from build123d import *

# Parameters (mm, degrees)
F0_W      = 50
F0_H      = 100
F1_DEPTH  = 20
F2_R      = 10
F3_DEPTH  = 10
F4_R      = 5
F5_DEPTH  = 10
F6_R      = 5
F7_DEPTH  = 10
F8_W      = 50
F8_H      = 10
F9_DEPTH  = 110
F10_R     = 10
F12_DEPTH = 10


with BuildPart() as f1:
    # F0 (on Top) → F1 (new body)
    with BuildSketch(Plane.XY):
        with Locations((25, 50)):
            Rectangle(F0_W, F0_H)
    extrude(amount=F1_DEPTH)

    # F2 (on face) → F3 (cut)
    with BuildSketch(Plane.XY.offset(20)):
        with Locations((25, 75)):
            Circle(F2_R)
        with Locations((25, 40)):
            Circle(F2_R)
    extrude(amount=-F3_DEPTH, mode=Mode.SUBTRACT)

    # F4 (on face) → F5 (cut)
    with BuildSketch(Plane.XY.offset(10)):
        with Locations((25, 75)):
            Circle(F4_R)
    extrude(amount=-F5_DEPTH, mode=Mode.SUBTRACT)

    # F6 (on face) → F7 (cut)
    with BuildSketch(Plane.XY.offset(10)):
        with Locations((25, 40)):
            Circle(F6_R)
    extrude(amount=-F7_DEPTH, mode=Mode.SUBTRACT)

    # F8 (on face) → F9 (join)
    with BuildSketch(Plane.XY.offset(20)):
        with Locations((25, 5)):
            Rectangle(F8_W, F8_H)
    extrude(amount=F9_DEPTH)

    # F10
    f10_edges = [f1.edges().sort_by_distance(p)[0] for p in [
        (0, 100, 10),
        (50, 100, 10),
        (0, 5, 130),
        (50, 5, 130),
    ]]
    fillet(f10_edges, radius=F10_R)

    # F11 (on face) → F12 (cut)
    with BuildSketch(Plane(origin=(0, 10, 0), x_dir=(-1, 0, 0), z_dir=(0, 1, 0))):
        with BuildLine():
            Line((-33, 105), (-33, 40))
            ThreePointArc((-33, 40), (-25, 32), (-17, 40))
            Line((-17, 40), (-17, 105))
            ThreePointArc((-17, 105), (-25, 113), (-33, 105))
        make_face()
    extrude(amount=-F12_DEPTH, mode=Mode.SUBTRACT)


solid = f1.part
Input: part model. Units: mm. Frame: model coordinates. A direction names the side the tool comes from. Give positions to 0.01 mm unless a question says otherwise; leave off trailing zeros. Write each loop counter-clockwise with the first axis right and the second up, starting at its lowest first coordinate (ties: lowest second). Pieces come first, ordered by that corner, then holes. Notation, with made-up numbers: (74, 18.25) -> (123, 18.25) arc R15 ccw to (123, 35.25) -> close; hole circle Ø1 at (56.5, -25.75). An arc over 180 degrees is marked (long way). Use one line per item in the form item = value. Start each with the question number.
1) Pin query (flat end, axial travel): pin 1 (1 mm diameter, centred on x = 31, z = 106, fed in from -Y); pin 2 (12 mm diameter, centred on x = 25, y = 40, fed in from +Z); pin 3 (4 mm diameter, centred on x = 35.5, z = 106.5, fed in from +Y); pin 4 (16 mm diameter, centred on x = 23.5, y = 77, fed in from +Z). Return the tip coordinate at first contact, or that it passes through.
2) Section query B-B on y = 40. Return the cut outline in (x, z).
3) Draft query along X for faces 5 (the cylindrical face through (25, 5, 113)), 6 (the cylindrical face through (47.15, 96.99, 10.14)), 7 (the cylindrical face through (2.85, 96.99, 10.14)). Return one class per face: pulls with the +X half, pulls with the -X half, needs draft (parallel to the pull), parting line crosses it, or undercut.
4) Set-up query: faces 1 (the flat face through (25, 56, 20)), 2 (the flat face through (20, 73, 10)), 3 (the flat face through (33, 5, 73)), 4 (the flat face through (25, 5, 130)). Return all of +Z, -Z, +X, -X, +Y, -Y with unobstructed straight access to the full face (end or side cutting, diameter ignored); none if empty.
5) Section query D-D on x = 8.5. Return the cut outline in (y, z), then the cut area to 3 significant figures.
6) Ray query, probe 1 along Y at (x, z) = (25, 14.75); probe 2 along Y at (x, z) = (25, 5); probe 3 along Z at (x, y) = (14, 63). Return the intervals inside material, ascending. Write a range as from..to.
7) Section query C-C on z = 16.5. Return the cut outline in (x, y).
8) Section query A-A on z = 90. Return the cut outline in (x, y).
Outcome:
q1.pin_1 = through
q1.pin_2 = 10
q1.pin_3 = 10
q1.pin_4 = 20
q2.outline = (0, 0) -> (20, 0) -> (20, 10) -> (15, 10) -> (15, 20) -> (0, 20) -> close; (30, 0) -> (50, 0) -> (50, 20) -> (35, 20) -> (35, 10) -> (30, 10) -> close
q3.face_5 = undercut
q3.face_6 = pulls with the +X half
q3.face_7 = pulls with the -X half
q4.face_1 = +Z, +X, -X, +Y
q4.face_2 = +Z
q4.face_3 = +Y, -Y
q4.face_4 = +Z, +X, -X, +Y, -Y
q5.outline = (0, 0) -> (99.89, 0) -> (99.89, 20) -> (10, 20) -> (10, 129.89) -> (0, 129.89) -> close
q5.area = 3,100 mm^2
q6.probe_1 = 0..30, 50..65, 85..100
q6.probe_2 = 0..35, 45..70, 80..100
q6.probe_3 = 0..20
q7.outline = (0, 0) -> (50, 0) -> (50, 90) arc R10 ccw to (40, 100) -> (10, 100) arc R10 ccw to (0, 90) -> close; hole circle Ø20 at (25, 40); hole circle Ø20 at (25, 75)
q8.outline = (0, 0) -> (17, 0) -> (17, 10) -> (0, 10) -> close; (33, 0) -> (50, 0) -> (50, 10) -> (33, 10) -> close
